Check sheet for the modelled part. Datum: model origin and axes. Units: mm. Face numbers are marked on the shaded views. A direction names the side the tool comes from. Give positions to 0.01 mm unless a question says otherwise; leave off trailing zeros. Write each loop counter-clockwise with the first axis right and the second up, starting at its lowest first coordinate (ties: lowest second). Pieces come first, ordered by that corner, then holes. Notation, with made-up numbers: (6, 10) -> (35, 10) arc R28 cw to (35, 31) -> close; hole circle Ø3 at (33, -24). An arc over 180 degrees is marked (long way). Return JSON: item names as keys, results as strings.
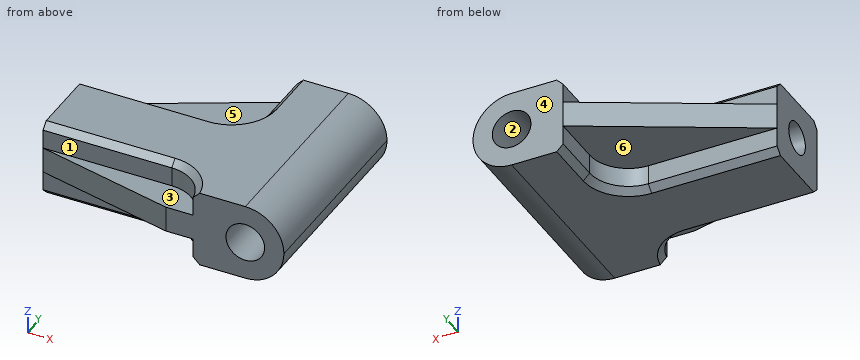
from build123d import *

# Parameters (mm, degrees)
SKETCH1_W               = 7
SKETCH1_H               = 6
BOSS_EXTRUDE1_DEPTH     = 16
FILLET1_R               = 3
SKETCH2_R               = 1.5
CUT_EXTRUDE1_DEPTH      = 16
SKETCH3_W               = 6
SKETCH3_H               = 6
BOSS_EXTRUDE2_DEPTH     = 13
FILLET2_R               = 3
CHAMFER1_SIZE           = 0.5
RIB1_REACH              = 25.179
SKETCH6_WALL_W          = 63.122131006
SKETCH6_WALL_H          = 2
RIB6_REACH              = 25.179
SKETCH7_WALL_W          = 61.69897201
SKETCH7_WALL_H          = 2
SKETCH8_R               = 1.25
CUT_EXTRUDE4_DEPTH      = 15
CUT_EXTRUDE6_DEPTH      = 24.178653973
CUT_EXTRUDE6_DEPTH_BACK = 24.178653973
SKETCH10_W              = 6
SKETCH10_H              = 0.5


with BuildPart() as part:
    # Sketch1 → Boss-Extrude1 (new body)
    with BuildSketch(Plane(origin=(0, 0, 0), x_dir=(1, 0, 0), z_dir=(0, 1, 0))):
        Rectangle(SKETCH1_W, SKETCH1_H)
    extrude(amount=BOSS_EXTRUDE1_DEPTH)

    # Fillet1
    fillet1_edges = [part.edges().sort_by_distance(p)[0] for p in [
        (3.5, 8, 3),
        (3.5, 8, -3),
    ]]
    fillet(fillet1_edges, radius=FILLET1_R - 0.0001)  # a hair under: the kernel refuses the full size

    # Sketch2 → Cut-Extrude1 (cut)
    with BuildSketch(Plane(origin=(0, 16, 0), x_dir=(1, 0, 0), z_dir=(0, 1, 0))):
        with Locations(Location((0.5, 0, 0), (0, 0, 270))):
            Circle(SKETCH2_R)
    extrude(amount=-CUT_EXTRUDE1_DEPTH, mode=Mode.SUBTRACT)

    # Sketch3 → Boss-Extrude2 (add)
    with BuildSketch(Plane.ZY.offset(3.5)):
        with Locations((0, 6)):
            Rectangle(SKETCH3_W, SKETCH3_H)
    extrude(amount=BOSS_EXTRUDE2_DEPTH)

    # Fillet2
    fillet2_edges = [part.edges().sort_by_distance(p)[0] for p in [
        (-3.5, 3, 0),
        (-3.5, 9, 0),
    ]]
    fillet(fillet2_edges, radius=FILLET2_R - 0.0001)  # a hair under: the kernel refuses the full size

    # Chamfer1
    chamfer1_edges = [part.edges().sort_by_distance(p)[0] for p in [
        (-11.49995, 9, -3),
        (-11.49995, 3, -3),
        (-11.49995, 3, 3),
        (-11.49995, 9, 3),
        (-4.378650367, 9.878650367, -3),
        (-4.378650367, 9.878650367, 3),
        (-4.378650367, 2.121349633, 3),
        (-4.378650367, 2.121349633, -3),
        (-3.5, 13.99995, 3),
        (-3.5, 13.99995, -3),
    ]]
    chamfer(chamfer1_edges, length=CHAMFER1_SIZE)

    # Sketch6 wall → Rib1 (add, up to next)
    with BuildSketch(Plane(origin=(-10, 12.5, 0), x_dir=(-0.880471099922, -0.474099823035, 0), z_dir=(-0.474099823035, 0.880471099922, 0)), mode=Mode.PRIVATE) as rib1_sk1:
        Rectangle(SKETCH6_WALL_W, SKETCH6_WALL_H)
    rib1_tool1 = extrude(rib1_sk1.sketch, amount=-RIB1_REACH, mode=Mode.PRIVATE) - part.part
    add(rib1_tool1.solids().sort_by_distance((-10, 12.5, 0))[0])

    # Sketch7 wall → Rib6 (add, up to next)
    with BuildSketch(Plane(origin=(-10, 1.5, 0), x_dir=(-0.974391195695, 0.224859506699, 0), z_dir=(0.224859506699, 0.974391195695, 0)), mode=Mode.PRIVATE) as rib6_sk1:
        Rectangle(SKETCH7_WALL_W, SKETCH7_WALL_H)
    rib6_tool1 = extrude(rib6_sk1.sketch, amount=RIB6_REACH, mode=Mode.PRIVATE) - part.part
    add(rib6_tool1.solids().sort_by_distance((-10, 1.5, 0))[0])

    # Sketch8 → Cut-Extrude4 (cut)
    with BuildSketch(Plane.ZY.offset(16.5)):
        with Locations((0, 6)):
            Circle(SKETCH8_R)
    extrude(amount=-CUT_EXTRUDE4_DEPTH, mode=Mode.SUBTRACT)

    # Sketch10 → Cut-Extrude6 (cut, two sides: drawn at the far end of the back side and taken through both)
    with BuildSketch(Plane(origin=(0, 0, 0), x_dir=(0, 0, -1), z_dir=(1, 0, 0)).offset(-CUT_EXTRUDE6_DEPTH_BACK)):
        with Locations((0, 0.25)):
            Rectangle(SKETCH10_W, SKETCH10_H)
    extrude(amount=CUT_EXTRUDE6_DEPTH + CUT_EXTRUDE6_DEPTH_BACK, mode=Mode.SUBTRACT)


solid = part.part
(1) Depth check by flat-ended pin: pin 1 Ø0.8 at (y, z) = (14, 2) entering from -X; pin 2 Ø2 at (x, y) = (-9.5, 1.5) entering from -Z; pin 3 Ø2 at (x, y) = (-12.5, 11.5) entering from +Z. Enter the tip coordinate at first touch or a pass-through.
Reply:
{"pin 1": "x = -3.5", "pin 2": "z = -1", "pin 3": "z = 1"}
(2) Cross-section at B-B on z = -0.25. Enter the section's corners in (x, y), then the cut area to 3 significant figures.
Reply:
{"outline": "(-16.5, 3) -> (-5.67, 0.5) -> (-0.98, 0.5) -> (-0.98, 16) -> (-3.5, 16) -> (-16.5, 9) -> (-16.5, 7.22) -> (-1.5, 7.22) -> (-1.5, 4.78) -> (-16.5, 4.78) -> close; (1.98, 0.5) -> (3.49, 0.5) -> (3.49, 16) -> (1.98, 16) -> close", "area": "168 mm^2"}
(3) Thickness scan on L1, parallel to Y at x = -2.25, z = 0; L2, parallel to X at y = 8.25, z = 0; L3, parallel to Y at x = -8, z = -2. Record the ranges inside material, lowest first.
Reply:
{"L1": "0.5 to 4.75, 7.25 to 16", "L2": "-16.5 to -1, 2 to 3.5", "L3": "3 to 9"}
(4) Release check for a two-part mould opening along Z. For the marked faces 1, 2 and 3 record: pulls with the +Z half, pulls with the -Z half, needs draft (parallel to the pull), parting line crosses it, or undercut.
Reply:
{"face 1": "needs draft", "face 2": "undercut", "face 3": "pulls with the +Z half"}
(5) Cross-section at C-C on x = 0. Enter the section's corners in (y, z).
Reply:
{"outline": "(0.5, -3) -> (16, -3) -> (16, -1.41) -> (0.5, -1.41) -> close; (0.5, 1.41) -> (16, 1.41) -> (16, 3) -> (0.5, 3) -> close"}
(6) Set-up check for the marked faces 4, 5 and 6: record each of +Z, -Z, +X, -X, +Y, -Y from which the full face is reachable in a straight line by a thin tool's end or side.
Reply:
{"face 4": "+Z, -Z, +X, -X, +Y", "face 5": "+Z, -X, +Y", "face 6": "-Z, -X, +Y"}
(7) Cross-section at D-D on x = -8. Enter the section's corners in (y, z), then the cut area to 3 significant figures.
Reply:
{"outline": "(1.04, -1) -> (3, -1) -> (3, -2.5) -> (3.5, -3) -> (8.5, -3) -> (9, -2.5) -> (9, -1) -> (13.58, -1) -> (13.58, 1) -> (9, 1) -> (9, 2.5) -> (8.5, 3) -> (3.5, 3) -> (3, 2.5) -> (3, 1) -> (1.04, 1) -> close; hole circle Ø2.5 at (6, 0)", "area": "43.7 mm^2"}
